```python
from build123d import *

# Parameters (mm, degrees)
BOSS_EXTRU_1_DEPTH       = 3
CONG_1_R                 = 20
CONG_2_R                 = 5
BOSS_EXTRU_2_DEPTH       = 5
CONG_4_R                 = 2
CONG_5_R                 = 4
ESQUISSE3_R              = 1.5
ENL_V_MAT_EXTRU_2_DEPTH  = 25
ESQUISSE4_R              = 1.7
ENL_V_MAT_EXTRU_3_DEPTH  = 25
ESQUISSE5_R              = 1.7
ENL_V_MAT_EXTRU_4_DEPTH  = 10
ESQUISSE6_R              = 1.7
ENL_V_MAT_EXTRU_5_DEPTH  = 10
CONG_6_R                 = 10
ENL_V_MAT_EXTRU_8_DEPTH  = 10
ESQUISSE8_R              = 1.5
ESQUISSE8_W              = 30
ESQUISSE8_H              = 2
ENL_V_MAT_EXTRU_10_DEPTH = 10
BOSS_EXTRU_3_START       = 3
ESQUISSE8_3_R            = 3.5
ESQUISSE8_3_R_2          = 1.5
BOSS_EXTRU_3_DEPTH       = 3
ENL_V_MAT_EXTRU_11_DEPTH = 6.5


with BuildPart() as part:
    # Esquisse1 → Boss.-Extru.1 (new body)
    with BuildSketch(Plane(origin=(0, 0, 0), x_dir=(1, 0, 0), z_dir=(0, 1, 0))):
        with BuildLine():
            Line((-37.5, 95), (37.5, 95))
            Line((37.5, 95), (37.5, 51))
            Line((37.5, 51), (44.874265815, 49.29751659))
            ThreePointArc((44.874265815, 49.29751659), (53.239122353, 44.019685168), (56.5, 34.681965619))
            Line((56.5, 34.681965619), (56.5, -26.800001164))
            ThreePointArc((56.5, -26.800001164), (52.990666647, -36.441815309), (44.104722665, -41.572117459))
            Line((44.104722665, -41.572117459), (17, -46.351411369))
            Line((17, -46.351411369), (17, -61.9))
            Line((17, -61.9), (27, -61.9))
            Line((27, -61.9), (27, -66.9))
            Line((27, -66.9), (17, -66.9))
            Line((17, -66.9), (17, -79.1))
            Line((17, -79.1), (27, -79.1))
            Line((27, -79.1), (27, -84.1))
            Line((27, -84.1), (17, -84.1))
            Line((17, -84.1), (17, -95))
            Line((17, -95), (-17, -95))
            Line((-17, -95), (-17, -84.1))
            Line((-17, -84.1), (-27, -84.1))
            Line((-27, -84.1), (-27, -79.1))
            Line((-27, -79.1), (-17, -79.1))
            Line((-17, -79.1), (-17, -66.9))
            Line((-17, -66.9), (-27, -66.9))
            Line((-27, -66.9), (-27, -61.9))
            Line((-27, -61.9), (-17, -61.9))
            Line((-17, -61.9), (-17, -46.351411369))
            Line((-17, -46.351411369), (-44.104722665, -41.572117459))
            ThreePointArc((-44.104722665, -41.572117459), (-52.990666647, -36.441815309), (-56.5, -26.800001164))
            Line((-56.5, -26.800001164), (-56.5, 34.681965619))
            ThreePointArc((-56.5, 34.681965619), (-53.239122353, 44.019685168), (-44.874265815, 49.29751659))
            Line((-44.874265815, 49.29751659), (-37.5, 51))
            Line((-37.5, 51), (-37.5, 95))
        make_face()
    extrude(amount=BOSS_EXTRU_1_DEPTH)

    # Congé1
    # the kernel refuses this fillet: 20 mm, written as the material it adds along each edge
    with BuildSketch(Plane(origin=(17, 0, 46.351411369), x_dir=(0.9848077530122094, 0, -0.1736481776669235), z_dir=(0, 1, 0))) as cong_1_piece_1:
        with BuildLine():
            CenterArc((16.742910017, -20), CONG_1_R, 90, 76.444834731)
            Line((-2.699984081, -15.312370632), (-3.088841963, -15.218618044))
            ThreePointArc((-3.088841963, -15.218618044), (-1.743915142, -7.586726045), (-0.393923101, 0.069459271))
            Line((-0.393923101, 0.069459271), (0, 0.4))
            Line((0, 0.4), (16.742910017, 0.4))
            Line((16.742910017, 0.4), (16.742910017, 0))
        make_face()
    extrude(amount=3)
    with BuildSketch(Plane(origin=(-17, 0, 46.351411369), x_dir=(0, 0, 1), z_dir=(0, 1, 0))) as cong_1_piece_2:
        with BuildLine():
            CenterArc((16.788779247, -19.961511146), CONG_1_R, 93.555165269, 76.444834731)
            Line((-2.907375813, -16.488547593), (-3.301298915, -16.419088322))
            Line((-3.301298915, -16.419088322), (-0.393923101, 0.069459271))
            Line((-0.393923101, 0.069459271), (0, 0.4))
            ThreePointArc((0, 0.4), (7.774294315, 0.4), (15.523784818, 0.399230223))
            Line((15.523784818, 0.399230223), (15.548588631, 0))
        make_face()
    extrude(amount=3)

    # Congé2
    cong_2_edges = [part.edges().sort_by_distance(p)[0] for p in [
        (-17, 1.5, 61.9),
        (17, 1.5, 61.9),
    ]]
    fillet(cong_2_edges, radius=CONG_2_R)

    # Esquisse2 → Boss.-Extru.2 (add)
    with BuildSketch(Plane.XY.offset(84.1)):
        Polygon((-27, 5), (-27, 8.904402326), (-16.833134842, 8.904402326), (-14.427579086, 3), (-14.427579086, 0), (-27, 0), align=None)
        Polygon((16.833134842, 8.904402326), (14.427579086, 3), (14.427579086, 0), (27, 0), (27, 5), (27, 8.904402326), align=None)
    boss_extru_2 = extrude(amount=-BOSS_EXTRU_2_DEPTH)

    # Symétrie1: Boss.-Extru.2 across plane
    add(boss_extru_2.mirror(Plane.XY.offset(73)))

    # Congé4
    cong_4_edges = [part.edges().sort_by_distance(p)[0] for p in [
        (16.833134842, 8.904402326, 81.6),
        (14.427579086, 3, 81.6),
        (-16.833134842, 8.904402326, 81.6),
        (-14.427579086, 3, 81.6),
        (16.833134842, 8.904402326, 64.4),
        (14.427579086, 3, 64.4),
        (-14.427579086, 3, 64.4),
        (-16.833134842, 8.904402326, 64.4),
    ]]
    fillet(cong_4_edges, radius=CONG_4_R)

    # Congé5
    cong_5_edges = [part.edges().sort_by_distance(p)[0] for p in [
        (27, 8.904402326, 81.6),
        (-27, 8.904402326, 81.6),
        (27, 8.904402326, 64.4),
        (-27, 8.904402326, 64.4),
        (-27, 0, 64.4),
        (-27, 0, 81.6),
        (27, 0, 81.6),
        (27, 0, 64.4),
    ]]
    fillet(cong_5_edges, radius=CONG_5_R)

    # Esquisse3 → Enlèv. mat.-Extru.2 (cut)
    with BuildSketch(Plane.XY.offset(84.1)):
        with Locations((-22, 4.452201163)):
            Circle(ESQUISSE3_R)
        with Locations(Location((22, 4.452201163, 0), (0, 0, 284.503100137))):
            Circle(ESQUISSE3_R)
    extrude(amount=-ENL_V_MAT_EXTRU_2_DEPTH, mode=Mode.SUBTRACT)

    # Esquisse4 → Enlèv. mat.-Extru.3 (cut)
    with BuildSketch(Plane(origin=(0, 3, 0), x_dir=(1, 0, 0), z_dir=(0, 1, 0))):
        with Locations(Location((-10, -90.8, 0), (0, 0, 270))):
            Circle(ESQUISSE4_R)
        with Locations(Location((10, -90.8, 0), (0, 0, 270))):
            Circle(ESQUISSE4_R)
        with Locations(Location((8.90673672, -64.828011588, 0), (0, 0, 270))):
            Circle(ESQUISSE4_R)
        with Locations(Location((8.90673672, -81.171988412, 0), (0, 0, 270))):
            Circle(ESQUISSE4_R)
        with Locations(Location((-8.90673672, -81.171988412, 0), (0, 0, 270))):
            Circle(ESQUISSE4_R)
        with Locations(Location((-8.90673672, -64.828011588, 0), (0, 0, 270))):
            Circle(ESQUISSE4_R)
    extrude(amount=-ENL_V_MAT_EXTRU_3_DEPTH, mode=Mode.SUBTRACT)

    # Esquisse5 → Enlèv. mat.-Extru.4 (cut)
    with BuildSketch(Plane(origin=(0, 3, 0), x_dir=(1, 0, 0), z_dir=(0, 1, 0))):
        with Locations(Location((15.5, 83, 0), (0, 0, 270))):
            Circle(ESQUISSE5_R)
        with Locations(Location((15.5, 49, 0), (0, 0, 270))):
            Circle(ESQUISSE5_R)
        with Locations(Location((-13, 83, 0), (0, 0, 270))):
            Circle(ESQUISSE5_R)
        with Locations(Location((-13, 67, 0), (0, 0, 270))):
            Circle(ESQUISSE5_R)
        with Locations(Location((27.5, 80, 0), (0, 0, 270))):
            Circle(ESQUISSE5_R)
        with Locations(Location((27.5, 55, 0), (0, 0, 270))):
            Circle(ESQUISSE5_R)
        with Locations(Location((27.5, 89, 0), (0, 0, 270))):
            Circle(ESQUISSE5_R)
        with Locations(Location((-27.5, 89, 0), (0, 0, 270))):
            Circle(ESQUISSE5_R)
        with Locations(Location((-27.5, 80, 0), (0, 0, 270))):
            Circle(ESQUISSE5_R)
        with Locations(Location((-27.5, 55, 0), (0, 0, 270))):
            Circle(ESQUISSE5_R)
        with Locations(Location((0, 89, 0), (0, 0, 270))):
            Circle(ESQUISSE5_R)
    extrude(amount=-ENL_V_MAT_EXTRU_4_DEPTH, mode=Mode.SUBTRACT)

    # Esquisse6 → Enlèv. mat.-Extru.5 (cut)
    with BuildSketch(Plane(origin=(0, 3, 0), x_dir=(1, 0, 0), z_dir=(0, 1, 0))):
        with Locations(Location((-52.484739006, 32.940982227, 0), (0, 0, 270))):
            Circle(ESQUISSE6_R)
        with Locations(Location((-52.484739006, -25.059017773, 0), (0, 0, 270))):
            Circle(ESQUISSE6_R)
        with Locations(Location((52.484739006, -25.059017773, 0), (0, 0, 90))):
            Circle(ESQUISSE6_R)
        with Locations(Location((52.484739006, 32.940982227, 0), (0, 0, 90))):
            Circle(ESQUISSE6_R)
    extrude(amount=-ENL_V_MAT_EXTRU_5_DEPTH, mode=Mode.SUBTRACT)

    # Congé6
    cong_6_edges = [part.edges().sort_by_distance(p)[0] for p in [
        (37.5, 1.5, -95),
        (-37.5, 1.5, -95),
    ]]
    fillet(cong_6_edges, radius=CONG_6_R)

    # Esquisse7 → Enlèv. mat.-Extru.8 (cut, symmetric)
    with BuildSketch(Plane(origin=(0, 3, 0), x_dir=(1, 0, 0), z_dir=(0, 1, 0))):
        Polygon((-86.454887478, 51), (-37.5, 51), (-37.5, 40), (20.5, 40), (20.5, 51), (91.524772855, 51), (68.271042048, 103.22710764), (-47.050718145, 103.22710764), align=None)
        Polygon((-33.488547593, -43.444035556), (33.488547593, -43.444035556), (53.128015595, -56.162105977), (47.497778975, -107.906661581), (-41.245474419, -107.906661581), (-59.476716808, -77.074413423), align=None)
    extrude(amount=ENL_V_MAT_EXTRU_8_DEPTH, both=True, mode=Mode.SUBTRACT)

    # Esquisse8 → Enlèv. mat.-Extru.10 (cut, symmetric)
    with BuildSketch(Plane(origin=(0, 3, 0), x_dir=(1, 0, 0), z_dir=(0, 1, 0))):
        with Locations(Location((41.5, 36.5, 0), (0, 0, 90))):
            Circle(ESQUISSE8_R)
        with Locations((7.26572134, -17)):
            Rectangle(ESQUISSE8_W, ESQUISSE8_H)
        with Locations(Location((-16.5, -12.5, 0), (0, 0, 90))):
            Circle(ESQUISSE8_R)
        with Locations(Location((-16.5, 36.5, 0), (0, 0, 90))):
            Circle(ESQUISSE8_R)
        with Locations(Location((41.5, -12.5, 0), (0, 0, 90))):
            Circle(ESQUISSE8_R)
    extrude(amount=ENL_V_MAT_EXTRU_10_DEPTH, both=True, mode=Mode.SUBTRACT)

    # Esquisse8<3> → Boss.-Extru.3 (add)
    # profile 1 of 4: a face of its own
    with BuildSketch(Plane(origin=(0, 3, 0), x_dir=(1, 0, 0), z_dir=(0, 1, 0)).offset(BOSS_EXTRU_3_START)):
        with Locations(Location((-16.5, -12.5, 0), (0, 0, 90))):
            Circle(ESQUISSE8_3_R)
        with Locations(Location((-16.5, -12.5, 0), (0, 0, 270))):
            Circle(ESQUISSE8_3_R_2, mode=Mode.SUBTRACT)
    # profile 2 of 4: a face of its own
    with BuildSketch(Plane(origin=(0, 3, 0), x_dir=(1, 0, 0), z_dir=(0, 1, 0)).offset(BOSS_EXTRU_3_START)):
        with Locations(Location((41.5, -12.5, 0), (0, 0, 90))):
            Circle(ESQUISSE8_3_R)
        with Locations(Location((41.5, -12.5, 0), (0, 0, 270))):
            Circle(ESQUISSE8_3_R_2, mode=Mode.SUBTRACT)
    # profile 3 of 4: a face of its own
    with BuildSketch(Plane(origin=(0, 3, 0), x_dir=(1, 0, 0), z_dir=(0, 1, 0)).offset(BOSS_EXTRU_3_START)):
        with Locations(Location((41.5, 36.5, 0), (0, 0, 90))):
            Circle(ESQUISSE8_3_R)
        with Locations(Location((41.5, 36.5, 0), (0, 0, 270))):
            Circle(ESQUISSE8_3_R_2, mode=Mode.SUBTRACT)
    # profile 4 of 4: a face of its own
    with BuildSketch(Plane(origin=(0, 3, 0), x_dir=(1, 0, 0), z_dir=(0, 1, 0)).offset(BOSS_EXTRU_3_START)):
        with Locations(Location((-16.5, 36.5, 0), (0, 0, 90))):
            Circle(ESQUISSE8_3_R)
        with Locations(Location((-16.5, 36.5, 0), (0, 0, 270))):
            Circle(ESQUISSE8_3_R_2, mode=Mode.SUBTRACT)
    extrude(amount=-BOSS_EXTRU_3_DEPTH)

    # Esquisse10 → Enlèv. mat.-Extru.11 (cut, symmetric)
    with BuildSketch(Plane(origin=(0, 3, 0), x_dir=(1, 0, 0), z_dir=(0, 1, 0))):
        with BuildLine():
            Line((-24.9, -36), (-24.9, -29))
            ThreePointArc((-24.9, -29), (-23.4, -27.5), (-21.9, -29))
            Line((-21.9, -29), (-21.9, -36))
            ThreePointArc((-21.9, -36), (-23.4, -37.5), (-24.9, -36))
        make_face()
        with BuildLine():
            Line((24.9, -36), (24.9, -29))
            ThreePointArc((24.9, -29), (23.4, -27.5), (21.9, -29))
            Line((21.9, -29), (21.9, -36))
            ThreePointArc((21.9, -36), (23.4, -37.5), (24.9, -36))
        make_face()
    extrude(amount=ENL_V_MAT_EXTRU_11_DEPTH, both=True, mode=Mode.SUBTRACT)


solid = part.part
```
Model file for the job. Use its own axes, mm. A direction names the side the tool comes from. Coordinates: 2 decimals unless noted, no trailing zeros. Order: outer loops, then holes, each group sorted by start corner. A loop starts at its lowest first (then second) coordinate and runs counter-clockwise, first axis right, second up. Notation, with made-up numbers: M 65,-32.75 L 74,-32.75 A30 cw 74,6.25 Z; hole C 19.25,85 d11. An arc over 180 degrees is marked long. Answer as CSV lines item,"result".
(1) Band-saw the part on C-C, the plane z = 31. List the corners of the cut face in (x, y).
Geometry says:
outline,"M -55.9,0 L -24.9,0 L -24.9,3 L -55.9,3 Z; M -21.9,0 L 21.9,0 L 21.9,3 L -21.9,3 Z; M 24.9,0 L 55.9,0 L 55.9,3 L 24.9,3 Z"
(2) Band-saw the part on B-B, the plane x = -23.4. List the corners of the cut face in (y, z), then the cut area to 3 significant figures.
Geometry says:
outline,"M 0,-40 L 3,-40 L 3,27.5 L 0,27.5 Z; M 0,37.5 L 3,37.5 L 3,43.44 L 0,43.44 Z"
area,"220 mm2"
(3) Pull direction Z, two halves, no side cores. Call faces 4 (the cylindrical face through (51.336, 1.521, 26.312)), 5 (the cylindrical face through (-52.9, 1.48, 36.55)), 6 (the cylindrical face through (53.15, 1.48, -44.13)): +Z half, -Z half, draft (parallel to the pull), parting line (faces both ways), or undercut.
Geometry says:
face 4,"undercut"
face 5,"+Z half"
face 6,"-Z half"
(4) Band-saw the part on D-D, the plane x = -47. List the corners of the cut face in (y, z), then the cut area to 3 significant figures.
Geometry says:
outline,"M 0,-48.64 L 3,-48.64 L 3,40.76 L 0,40.76 Z"
area,"268 mm2"
(5) 3-axis set-ups, long thin cutter, end or side, ignore diameter. For faces 1 (the flat face through (43, 6, -37.2)), 2 (the cylindrical face through (-23.4, 1.5, 27.5)), 3 (the cylindrical face through (38.03, 4.52, -36.04)): which of +Z, -Z, +X, -X, +Y, -Y reach the whole face in a straight line?
Geometry says:
face 1,"+Z, -Z, +X, -X, +Y"
face 2,"+Y, -Y"
face 3,"+Y"
(6) Flat gauge pins, fed straight in: pin 1 (5.5 mm diameter, centred on x = -52.48, z = -32.94, fed in from +Y); pin 2 (3 mm diameter, centred on x = 9, y = 3.5, fed in from -Z); pin 3 (2.5 mm diameter, centred on y = 2, z = -47, fed in from -X). Where does each tip first touch, or does it go through?
Geometry says:
pin 1,"stops at y = 3"
pin 2,"stops at z = -40"
pin 3,"stops at x = -51.62"
(7) Band-saw the part on A-A, the plane z = 12.5. List the corners of the cut face in (x, y), then the cut area to 3 significant figures.
Geometry says:
outline,"M -56.5,0 L -18,0 L -18,6 L -20,6 L -20,3 L -56.5,3 Z; M -15,0 L 40,0 L 40,6 L 38,6 L 38,3 L -13,3 L -13,6 L -15,6 Z; M 43,0 L 56.5,0 L 56.5,3 L 45,3 L 45,6 L 43,6 Z"
area,"345 mm2"
(8) Wall check: line 1 along Z through (x, y) = (41.5, 4.7); line 2 along Z through (x, y) = (11.5, 2.35); line 3 along Z through (x, y) = (41.5, 0.75). Give the ranges that are in metal, low to high.
Geometry says:
line 1,"z = -40 to -38, -35 to -33, 9 to 11, 14 to 16"
line 2,"z = -40 to 16, 18 to 43.44"
line 3,"z = -50.08 to -38, -35 to 11, 14 to 42.03"
